Source: CAD feature listing. Evaluate the final solid. Frame: model axes, mm. Face numbers are marked on the shaded views. A direction names the side the tool comes from. Coordinates: 2 decimals unless noted, no trailing zeros. Loops run counter-clockwise (first coordinate to the right, second up) from the corner with the lowest first, then second, coordinate; pieces in that order, holes last.
Item 1: Pull-direction query (X, two-part tool) for the marked faces 4, 5, 6 and 7; classes: +X half, -X half, draft (parallel to the pull), parting line (faces both ways), or undercut.
Item 2: Section query D-D, the plane y = -13.5. State how many separate pieces and enclosed holes the cut face has, then the cut area to 3 significant figures.
Item 3: Line query: probe 1 along Z at (x, y) = (-1, -13.75); probe 2 along X at (y, z) = (-13.25, 2); probe 3 along X at (y, z) = (1, -0.05). Output: solid intervals per line, ascending.
Item 4: Section query B-B, the plane y = 5. Return the cut outline in (x, z).
Item 5: Section query A-A, the plane x = 0. Return the cut outline in (y, z), then the cut area to 3 significant figures.
Item 6: Section query C-C, the plane z = -0.3. Return the cut outline in (x, y), then the cut area to 3 significant figures.
Item 7: Pin query (flat end, axial travel): pin 1 Ø2 at (x, y) = (0, -13.25) entering from -Z; pin 2 Ø1.1 at (x, y) = (0, -13.25) entering from +Z (1 decimal); pin 3 Ø1.5 at (x, y) = (1, -5) entering from -Z. Return the tip coordinate at first contact, or that it passes through.
Item 8: Reachability of the marked faces 1, 2 and 3 from +Z, -Z, +X, -X, +Y, -Y: full face, straight path, thin tool, end or side. Return the list, or none.
Solid Edge part; units mm, degrees
sketch "Sketch1" plane through (0, 0, 0) normal (0, -1, 0) x (1, 0, 0)
  circle A0 centre (0, 0) radius 1
extrude "Protrusion1" add sketch "Sketch1" along normal mid plane 16
sketch "Sketch2" plane through (0, -8, 0) normal (0, 0, -1) x (-1, 0, 0)
  circle A0 centre (0, -5.25) radius 0.95
  line L0 (2.125, 0) -> (2.4934, -5.0688)
  arc A1 (2.4934, -5.0688) -> (-2.4934, -5.0688) centre (0, -5.25) cw
  line L1 (-2.4934, -5.0688) -> (-2.125, 0)
  line L2 (-2.125, 0) -> (2.125, 0)
extrude "ExtrudedProtrusion_2" add sketch "Sketch2" along normal mid plane 5
sketch "Sketch3" plane through (2.3092, -10.5344, 0) normal (0.9973689, 0.0724935, 0) x (-0.0724935, 0.9973689, 0)
  line L0 (1.2911, -1.25) -> (-5.2803, -1.25)
  line L1 (-5.2803, -1.25) -> (-5.2803, 1.25)
  line L2 (-5.2803, 1.25) -> (1.2911, 1.25)
  line L3 (1.2911, 1.25) -> (1.2911, -1.25)
extrude "Cutout1" cut sketch "Sketch3" along normal through all and the other way through all
fillet "Round_1" radius 1 2 edges at (0, -8, -2.5) (0, -8, 2.5)
fillet "Round_1" radius 0.25 15 edges at (-2.3092, -10.5344, -2.5) (0, -15.75, -2.5) (2.3092, -10.5344, -2.5) (-2.125, -8, 0) (-2.3092, -10.5344, 2.5) (0, -15.75, 2.5) (2.3092, -10.5344, 2.5) (2.125, -8, 0) (2.2156, -9.2467, 0) (2.3545, -11.1577, -1.25) (-2.3663, -11.3196, -1.25) (2.3545, -11.1577, 1.25) (0, -15.75, 1.25) (-2.3663, -11.3196, 1.25) (-2.2392, -9.5705, 0)
properties material "Steel"
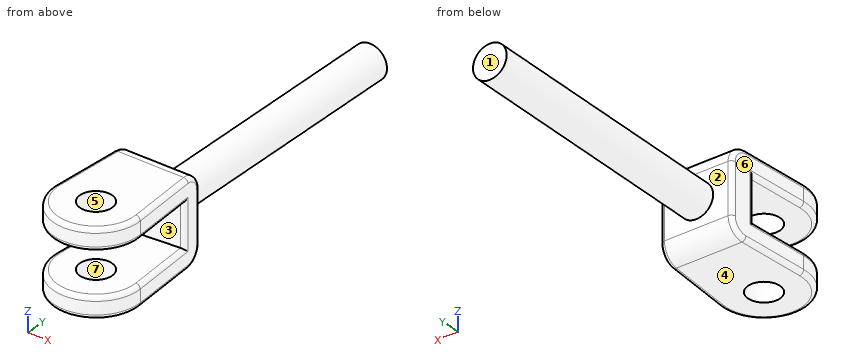
Verdict:
1. face 4: draft
1. face 5: undercut
1. face 6: -X half
1. face 7: undercut
2. separate pieces: 4
2. enclosed holes: 0
2. area: 7.75 mm2
3. probe 1: z = -2.5 to -1.25, 1.25 to 2.5
3. probe 2: x = -2.5 to -0.95, 0.95 to 2.5
3. probe 3: x = -1 to 1
4. outline: circle Ø2 at (0, 0)
5. outline: (-15.75, -2.25) arc R0.25 ccw to (-15.5, -2.5) - (-14.2, -2.5) - (-14.2, -1.25) - (-15.5, -1.25) arc R0.25 ccw to (-15.75, -1.5) - close; (-15.75, 1.5) arc R0.25 ccw to (-15.5, 1.25) - (-14.2, 1.25) - (-14.2, 2.5) - (-15.5, 2.5) arc R0.25 ccw to (-15.75, 2.25) - close; (-12.3, -2.5) - (-9, -2.5) arc R1 ccw to (-8, -1.5) - (-8, -1) - (8, -1) - (8, 1) - (-8, 1) - (-8, 1.5) arc R1 ccw to (-9, 2.5) - (-12.3, 2.5) - (-12.3, 1.25) - (-9.41, 1.25) - (-9.41, -1.25) - (-12.3, -1.25) - close
5. area: 49.7 mm2
6. outline: (-2.22, -9.28) arc R0.25 ccw to (-1.95, -9.55) - (1.97, -9.26) arc R0.25 ccw to (2.2, -9) - (2.14, -8.23) arc R0.25 ccw to (1.89, -8) - (0.95, -8) - (0.95, 8) - (-0.95, 8) - (-0.95, -8) - (-1.89, -8) arc R0.25 ccw to (-2.14, -8.23) - close
6. area: 36.6 mm2
7. pin 1: stops at z = -2.5
7. pin 2: passes through
7. pin 3: stops at z = -0.97
8. face 1: +Z, -Z, +X, -X, +Y
8. face 2: +Y
8. face 3: +X, -Y
